from build123d import *

# Parameters (mm, degrees)
F0_R     = 22.86
F1_DEPTH = 25.4
F2_R     = 31.75
F3_DEPTH = 12.7
F4_R     = 9.525
F5_DEPTH = 6.35


with BuildPart() as f1:
    # F0 (on Top) → F1 (new body)
    with BuildSketch(Plane.XY):
        Circle(F0_R)
    extrude(amount=F1_DEPTH)

    # F2 (on face) → F3 (join)
    with BuildSketch(Plane.XY.offset(25.4)):
        Circle(F2_R)
    extrude(amount=F3_DEPTH)

    # F4 (on Front) → F5 (join, symmetric)
    with BuildSketch(Plane.XZ):
        Polygon((-31.75, 38.1), (0, 38.1), (31.75, 38.1), (17.085303, 63.5), (0, 63.5), (-17.085303, 63.5), align=None)
        with Locations((0, 50.8)):
            Circle(F4_R, mode=Mode.SUBTRACT)
    extrude(amount=F5_DEPTH, both=True)


solid = f1.part
Can you work these out from the model? Positions are in its coordinate system, mm. A direction names the side the tool comes from. Coordinates: 2 decimals unless noted, no trailing zeros. Write each loop counter-clockwise with the first axis right and the second up, starting at its lowest first coordinate (ties: lowest second). Pieces come first, ordered by that corner, then holes. Notation, with made-up numbers: M -18.75,81.25 L 36.25,81.25 A20 cw 36.25,99.25 Z; hole C 53.25,27 d4. An arc over 180 degrees is marked long. Use one line per item in the form item = value.
Q1. I need wall thicknesses on line 1 along Z through (x, y) = (0, -3) (3 decimals); line 2 along Z through (x, y) = (-16, 21); line 3 along Y through (x, z) = (13.5, 52.5). Which ranges of each line are inside material? Lowest first, please. Write a range as from..to.
Model answer:
line_1 = 0..41.275, 60.325..63.5
line_2 = 25.4..38.1
line_3 = -6.35..6.35
Q2. For P1, Ø12.5, axis at x = -2, y = -25, coming from the +Z side; P2, Ø6, axis at x = 12, z = 50.5, coming from the +Y side; P3, Ø2, axis at x = -7.5, y = -25, coming from the -Z side, each with a flat end and sliding along its axis, tell me the tip position at first contact or that it passes through.
Model answer:
P1 = 38.1
P2 = 6.35
P3 = 25.4
Q3. We'd pull the mould along Z, two halves only. Please class faces 1 (the flat face through (24.52, -0.09, 50.62)), 2 (the cylindrical face through (21.804, 6.867, 12.522)), 3 (the cylindrical face through (-1.24, 0.089, 60.244)): +Z half, -Z half, draft (parallel to the pull), parting line (faces both ways), or undercut.
Model answer:
face_1 = +Z half
face_2 = draft
face_3 = undercut
Q4. If we section it at A-A (x = 0): Write out the boundary of the cut face in (y, z) (3 decimals).
Model answer:
outline = M -31.75,25.4 L -22.86,25.4 L -22.86,0 L 22.86,0 L 22.86,25.4 L 31.75,25.4 L 31.75,38.1 L 6.35,38.1 L 6.35,41.275 L -6.35,41.275 L -6.35,38.1 L -31.75,38.1 Z; M -6.35,60.325 L 6.35,60.325 L 6.35,63.5 L -6.35,63.5 Z
Q5. If we section it at D-D (z = 19): Write out the boundary of the cut face in (x, y), then the cut area to 3 significant figures.
Model answer:
outline = C 0,0 d45.72
area = 1,640 mm^2
Q6. For faces 4 (the flat face through (-8, 22, 25.4)), 5 (the flat face through (7, 6.35, 43)), 6 (the flat face through (0, 0, 63.5)), 7 (the flat face through (0, -16, 38.1)), which set-ups out of +Z, -Z, +X, -X, +Y, -Y let a thin tool reach every point of the face, with its end or its side?
Model answer:
face_4 = -Z
face_5 = +Z, +X, -X, +Y
face_6 = +Z, +X, -X, +Y, -Y
face_7 = +Z, +X, -X, -Y
Q7. If we section it at B-B (z = 55.5): Write out the boundary of the cut face in (x, y), then the cut area to 3 significant figures.
Model answer:
outline = M -21.7,-6.35 L -8.28,-6.35 L -8.28,6.35 L -21.7,6.35 Z; M 8.28,-6.35 L 21.7,-6.35 L 21.7,6.35 L 8.28,6.35 Z
area = 341 mm^2
Q8. If we section it at C-C (y = -12): Write out the boundary of the cut face in (x, z), then the cut area to 3 significant figures.
Model answer:
outline = M -29.39,25.4 L -19.46,25.4 L -19.46,0 L 19.46,0 L 19.46,25.4 L 29.39,25.4 L 29.39,38.1 L -29.39,38.1 Z
area = 1,740 mm^2
